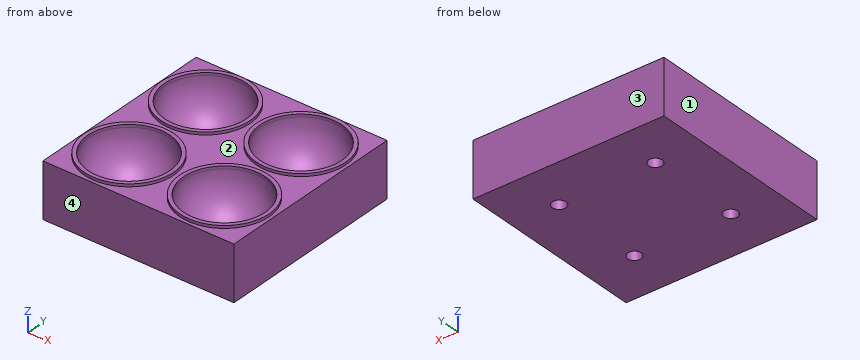
from build123d import *

# Parameters (mm, degrees)
F0_W     = 88.9
F0_H     = 88.9
F1_DEPTH = 50.8
F3_ANGLE = 180
F4_R     = 41.6097493144
F5_DEPTH = 2.54
F6_R     = 6.35
F7_DEPTH = 25.4


with BuildPart() as f1:
    # F0 (on Top) → F1 (new body)
    with BuildSketch(Plane.XY):
        with Locations((98.8394960349, 44.45)):
            Rectangle(F0_W, F0_H)
    extrude(amount=F1_DEPTH)

    # F2 (on face) → F3 (revolve, cut)
    with BuildSketch(Plane.XY.offset(50.8)):
        with BuildLine():
            ThreePointArc((60.7394960349, 44.45), (98.8394960349, 6.35), (136.9394960349, 44.45))
            Line((136.9394960349, 44.45), (60.7394960349, 44.45))
        make_face()
    revolve(axis=Axis((98.8394960349, 44.45, 50.8), (1, 0, 0)), revolution_arc=F3_ANGLE, mode=Mode.SUBTRACT)

    # F4 (on face) → F5 (join)
    with BuildSketch(Plane.XY.offset(50.8)):
        with Locations((98.8394960349, 44.45)):
            Circle(F4_R)
        with BuildLine():
            ThreePointArc((60.7394960349, 44.45), (98.8394960349, 82.55), (136.9394960349, 44.45))
            ThreePointArc((136.9394960349, 44.45), (98.8394960349, 6.35), (60.7394960349, 44.45))
        make_face(mode=Mode.SUBTRACT)
    extrude(amount=F5_DEPTH)

    # F6 (on face) → F7 (cut)
    with BuildSketch(Plane(origin=(0, 0, 0), x_dir=(1, 0, 0), z_dir=(0, 0, -1))):
        with Locations((99.2432538861, -43.760972516)):
            Circle(F6_R)
    extrude(amount=-F7_DEPTH, mode=Mode.SUBTRACT)

    # F8: F1 across face


with BuildPart() as f1_1:
    add(f1.part)
    add(f1.part.mirror(Plane(origin=(54.3894960349, 44.45, 25.4), x_dir=(0, -1, 0), z_dir=(-1, 0, 0))))

    # F9: F1 across face


with BuildPart() as f1_2:
    add(f1_1.part)
    add(f1_1.part.mirror(Plane(origin=(54.3894960349, 0, 25.4), x_dir=(1, 0, 0), z_dir=(0, -1, 0))))


solid = f1_2.part
Input: part model. Units: mm. Frame: model coordinates. Face numbers are marked on the shaded views. Give positions to 0.01 mm unless a question says otherwise; leave off trailing zeros. Order: outer loops, then holes, each group sorted by start corner. A loop starts at its lowest first (then second) coordinate and runs counter-clockwise, first axis right, second up.
Q1. Section B-B on z = 9. Output: boundary loops of the cut face in (x, y).
Checked values:
outline: (-34.51, -88.9) - (143.29, -88.9) - (143.29, 88.9) - (-34.51, 88.9) - close; hole circle Ø12.7 at (9.54, -43.76); hole circle Ø12.7 at (9.54, 43.76); hole circle Ø12.7 at (99.24, -43.76); hole circle Ø12.7 at (99.24, 43.76)
Q2. Section A-A on x = 8. Output: boundary loops of the cut face in (y, z).
Checked values:
outline: (-88.9, 0) - (-49.92, 0) - (-49.92, 13.14) arc R38.05 cw to (-82.5, 50.8) - (-82.5, 53.34) - (-86.01, 53.34) - (-86.01, 50.8) - (-88.9, 50.8) - close; (-37.6, 0) - (37.6, 0) - (37.6, 13.37) arc R38.05 cw to (6.4, 50.8) - (6.4, 53.34) - (2.89, 53.34) - (2.89, 50.8) - (-2.89, 50.8) - (-2.89, 53.34) - (-6.4, 53.34) - (-6.4, 50.8) arc R38.05 cw to (-37.6, 13.37) - close; (49.92, 0) - (88.9, 0) - (88.9, 50.8) - (86.01, 50.8) - (86.01, 53.34) - (82.5, 53.34) - (82.5, 50.8) arc R38.05 cw to (49.92, 13.14) - close
Q3. Draft query along Y for the marked faces 1, 2, 3 and 4. Return one class per face: +Y half, -Y half, draft (parallel to the pull), parting line (faces both ways), or undercut.
Checked values:
face 1: draft
face 2: undercut
face 3: +Y half
face 4: -Y half
Q4. Section C-C on y = 30.5. Output: boundary loops of the cut face in (x, z).
Checked values:
outline: (-34.51, 0) - (143.29, 0) - (143.29, 50.8) - (138.04, 50.8) - (138.04, 53.34) - (134.29, 53.34) - (134.29, 50.8) arc R35.45 cw to (63.39, 50.8) - (63.39, 53.34) - (59.64, 53.34) - (59.64, 50.8) - (49.14, 50.8) - (49.14, 53.34) - (45.39, 53.34) - (45.39, 50.8) arc R35.45 cw to (-25.51, 50.8) - (-25.51, 53.34) - (-29.26, 53.34) - (-29.26, 50.8) - (-34.51, 50.8) - close
Q5. Ray query, probe 1 along X at (y, z) = (-43.5, 6); probe 2 along X at (y, z) = (-44, 51); probe 3 along Y at (x, z) = (-4, 27). Return the intervals inside material, ascending.
Checked values:
probe 1: x = -34.51 to 3.19, 15.88 to 92.9, 105.59 to 143.29
probe 2: x = -31.67 to -28.16, 48.04 to 51.55, 57.23 to 60.74, 136.94 to 140.45
probe 3: y = -88.9 to -70.73, -18.17 to 18.17, 70.73 to 88.9
Q6. Contact query for flat-ended pins moving along their axis: pin 1 Ø16.5 at (x, y) = (99.24, 43.76) entering from +Z; pin 2 Ø20.5 at (x, y) = (99.24, -43.76) entering from +Z. Output: stop coordinate, or through.
Checked values:
pin 1: stops at z = 13.79
pin 2: stops at z = 14.34
Q7. Section D-D on x = 103. Output: boundary loops of the cut face in (y, z).
Checked values:
outline: (-88.9, 0) - (-48.88, 0) - (-48.88, 13.19) arc R37.87 cw to (-82.32, 50.8) - (-82.32, 53.34) - (-85.85, 53.34) - (-85.85, 50.8) - (-88.9, 50.8) - close; (-38.64, 0) - (38.64, 0) - (38.64, 13.38) arc R37.87 cw to (6.58, 50.8) - (6.58, 53.34) - (3.05, 53.34) - (3.05, 50.8) - (-3.05, 50.8) - (-3.05, 53.34) - (-6.58, 53.34) - (-6.58, 50.8) arc R37.87 cw to (-38.64, 13.38) - close; (48.88, 0) - (88.9, 0) - (88.9, 50.8) - (85.85, 50.8) - (85.85, 53.34) - (82.32, 53.34) - (82.32, 50.8) arc R37.87 cw to (48.88, 13.19) - close
